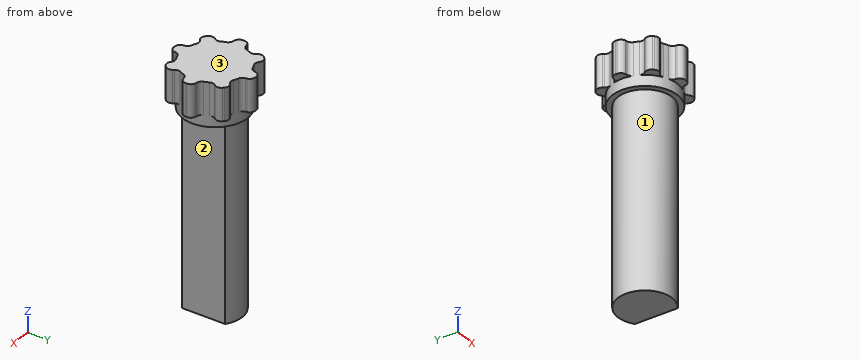
from build123d import *

# Parameters (mm, degrees)
BOSS_EXTRUDE1_DEPTH      = 25.4
SKETCH2_R                = 3.81
BOSS_EXTRUDE2_DEPTH      = 2.54
BOSS_EXTRUDE3_DEPTH      = 3.81
FILLET1_R                = 0.635
CIRPATTERN1_COUNT        = 8
FILLET1_OF_CIRPATTERN1_R = 0.635


with BuildPart() as part:
    # Sketch1 → Boss-Extrude1 (new body)
    with BuildSketch(Plane.XY):
        with BuildLine():
            Line((1.905, 2.54), (1.905, -2.54))
            ThreePointArc((1.905, -2.54), (-3.175, 0), (1.905, 2.54))
        make_face()
    extrude(amount=-BOSS_EXTRUDE1_DEPTH)

    # Sketch2 → Boss-Extrude2 (add, symmetric)
    with BuildSketch(Plane.XY):
        Circle(SKETCH2_R)
    extrude(amount=BOSS_EXTRUDE2_DEPTH, both=True)

    # Sketch4 → Boss-Extrude3 (add)
    with BuildSketch(Plane.XY.offset(2.54)):
        Polygon((-0.635, 4.826), (0.635, 4.826), (0.824634929, 3.719687787), (-0.824634929, 3.719687787), align=None)
    boss_extrude3 = extrude(amount=-BOSS_EXTRUDE3_DEPTH)

    # Fillet1
    fillet1_edges = [part.edges().sort_by_distance(p)[0] for p in [
        (0.635, 4.826, 0.635),
        (0.824634929, 3.719687787, 0.635),
        (-0.824634929, 3.719687787, 0.635),
        (-0.635, 4.826, 0.635),
    ]]
    fillet(fillet1_edges, radius=FILLET1_R)

    # CirPattern1: Boss-Extrude3 ×8 about axis
    cirpattern1_axis = Axis((0, 0, 0), (0, 0, 1))
    for i in range(1, CIRPATTERN1_COUNT):
        add(boss_extrude3.rotate(cirpattern1_axis, i * 360 / CIRPATTERN1_COUNT))

    # Fillet1 of CirPattern1
    fillet1_of_cirpattern1_edges = [part.edges().sort_by_distance(p)[0] for p in [
        (-2.96348452, 3.861510132, 0.635),
        (-2.047111508, 3.213321409, 0.635),
        (-3.213321409, 2.047111508, 0.635),
        (-3.861510132, 2.96348452, 0.635),
        (-4.826, 0.635, 0.635),
        (-3.719687787, 0.824634929, 0.635),
        (-3.719687787, -0.824634929, 0.635),
        (-4.826, -0.635, 0.635),
        (-3.861510132, -2.96348452, 0.635),
        (-3.213321409, -2.047111508, 0.635),
        (-2.047111508, -3.213321409, 0.635),
        (-2.96348452, -3.861510132, 0.635),
        (-0.635, -4.826, 0.635),
        (-0.824634929, -3.719687787, 0.635),
        (0.824634929, -3.719687787, 0.635),
        (0.635, -4.826, 0.635),
        (2.96348452, -3.861510132, 0.635),
        (2.047111508, -3.213321409, 0.635),
        (3.213321409, -2.047111508, 0.635),
        (3.861510132, -2.96348452, 0.635),
        (4.826, -0.635, 0.635),
        (3.719687787, -0.824634929, 0.635),
        (3.719687787, 0.824634929, 0.635),
        (4.826, 0.635, 0.635),
        (3.861510132, 2.96348452, 0.635),
        (3.213321409, 2.047111508, 0.635),
        (2.047111508, 3.213321409, 0.635),
        (2.96348452, 3.861510132, 0.635),
    ]]
    fillet(fillet1_of_cirpattern1_edges, radius=FILLET1_OF_CIRPATTERN1_R)


solid = part.part
Work out the finished part from the listing and answer in its coordinate system (mm). Face numbers are marked on the shaded views. A direction names the side the tool comes from. Give positions to 0.01 mm unless a question says otherwise; leave off trailing zeros. Write each loop counter-clockwise with the first axis right and the second up, starting at its lowest first coordinate (ties: lowest second). Pieces come first, ordered by that corner, then holes.
Q1. Straight lines are drawn through the part: L1, parallel to Z at x = -0.75, y = 4; L2, parallel to Z at x = 2.5, y = 2; L3, parallel to X at y = 0, z = -12 (3 decimals). For each, find the intervals that lie inside material, in ascending order.
Answer:
L1: z = -1.27 to 2.54
L2: z = -2.54 to 2.54
L3: x = -3.175 to 1.905
Q2. The part is cut by section B-B on z = -16.75. Give the vertices of the cut face in (x, y) (3 decimals), and give its area (3 significant figures).
Answer:
outline: (1.905, -2.54) - (1.905, 2.54) arc R3.175 ccw (long way) to start
area: 27.2 mm2
Q3. The part is cut by section A-A on y = 2. Give the vertices of the cut face in (x, z) (3 decimals), and give its area (3 significant figures).
Answer:
outline: (-3.33, -1.27) - (-3.243, -1.27) - (-3.243, -2.54) - (-2.466, -2.54) - (-2.466, -25.4) - (1.905, -25.4) - (1.905, -2.54) - (3.243, -2.54) - (3.243, -1.27) - (3.33, -1.27) - (3.33, 2.54) - (-3.33, 2.54) - close
area: 134 mm2
Q4. Given pin 1 (4 mm diameter, centred on y = 0, z = -14, fed in from +X) (3 decimals); pin 2 (1 mm diameter, centred on x = 2.5, y = -2.5, fed in from -Z); pin 3 (4 mm diameter, centred on x = 3, z = -12.5, fed in from +Y), each flat-ended and moving along its own axis, determine where each tip first touches the part or whether it passes through.
Answer:
pin 1: stops at x = 1.905
pin 2: stops at z = -2.54
pin 3: stops at y = 3.01
Q5. A tool of negligible diameter and unlimited length cuts with its end or side. For the marked faces 1, 2 and 3, from which of +Z, -Z, +X, -X, +Y, -Y can it reach the whole face along a straight path? Write none if from no direction.
Answer:
face 1: -Z
face 2: -Z, +X, +Y, -Y
face 3: +Z, +X, -X, +Y, -Y
